Autodesk Inventor part; units mm, degrees
ref_plane "YZ Plane" through (0, 0, 0) normal (1, 0, 0) x (0, 1, 0)
ref_plane "XZ Plane" through (0, 0, 0) normal (0, 1, 0) x (-1, 0, 0)
ref_plane "XY Plane" through (0, 0, 0) normal (0, 0, 1) x (1, 0, 0)
sketch "Sketch1" plane through (0, 0, 0) normal (0, 1, 0) x (-1, 0, 0)
  line L0 (13.5, 10) -> (-13.5, 10)
  line L1 (-13.5, 10) -> (-13.5, -10)
  line L2 (-13.5, -10) -> (13.5, -10)
  line L3 (13.5, -10) -> (13.5, 10)
  line L4 (13.5, 10) -> (-13.5, -10) construction
  line L5 (-13.5, 10) -> (13.5, -10) construction
  point P0 (0, 0)
  dimension "d0" = 27
  dimension "d1" = 20
extrude "Extrusion1" add sketch "Sketch1" along normal blind 3
sketch "Sketch2" plane through (0, 3, 0) normal (0, 1, 0) x (1, 0, 0)
  line L0 (-13.5, -10) -> (13.5, -10)
  line L1 (0, -10) -> (-10.5, -10)
  line L2 (-10.5, -10) -> (-10.5, -7)
  line L3 (-10.5, -7) -> (-10.5, 3.5)
  circle A0 centre (-10.5, -7) radius 1.25
  circle A1 centre (-10.5, 3.5) radius 1.25
  line L4 (-10.5, -7) -> (10.5, -7)
  line L5 (10.5, -7) -> (10.5, 3.5)
  circle A2 centre (10.5, -7) radius 1.25
  circle A3 centre (10.5, 3.5) radius 1.25
  point P0 (0, 0)
  dimension "d4" = 10.5
  dimension "d5" = 3
  dimension "d6" = 10.5
  dimension "d7" = 2.5
  dimension "d8" = 2.5
  dimension "d9" = 21
  dimension "d10" = 10.5
  dimension "d11" = 2.5
  dimension "d12" = 2.5
extrude "Extrusion2" cut sketch "Sketch2" against normal up to next
sketch "Sketch3" plane through (0, 0, 0) normal (0, -1, 0) x (1, 0, 0)
  line L0 (-13.5, 10) -> (13.5, 10)
  line L1 (0, 10) -> (0, 8.5)
  line L2 (7.5, 7) -> (-7.5, 7)
  line L3 (-7.5, 7) -> (-7.5, 10)
  line L4 (-7.5, 10) -> (7.5, 10)
  line L5 (7.5, 10) -> (7.5, 7)
  line L6 (7.5, 7) -> (-7.5, 10) construction
  line L7 (-7.5, 7) -> (7.5, 10) construction
  point P0 (0, 0)
  dimension "d15" = 1.5
  dimension "d16" = 15
  dimension "d17" = 3
extrude "Extrusion3" add sketch "Sketch3" along normal blind 8
sketch "Sketch4" plane through (7.5, 0, 7) normal (0, 0, -1) x (-1, 0, 0)
  circle A0 centre (3, -5) radius 1.25
  circle A1 centre (12, -5) radius 1.25
  line L0 (0, 0) -> (0, -8)
  line L1 (15, -8) -> (0, -8)
  line L2 (15, 0) -> (15, -8)
  point P0 (7.5, 0)
  dimension "d20" = 2.5
  dimension "d21" = 2.5
  dimension "d22" = 3
  dimension "d23" = 3
  dimension "d24" = 3
  dimension "d25" = 3
extrude "Extrusion4" cut sketch "Sketch4" against normal up to next
sketch "Sketch5" plane through (0, 0, 0) normal (0, -1, 0) x (1, 0, 0)
  line L0 (13.5, -10) -> (-13.5, -10)
  line L1 (13.5, -10) -> (7.5, -10)
  line L2 (7.5, -10) -> (-7.5, -10)
  line L3 (-7.5, -10) -> (-7.5, 7)
  line L4 (-7.5, 7) -> (7.5, 7)
  line L5 (7.5, 7) -> (7.5, -10)
  point P0 (0, 0)
  dimension "d28" = 6
extrude "Extrusion5" cut sketch "Sketch5" against normal up to next
fillet "Fillet1" radius 5 2 edges at (-7.5, 1.5, 7) (7.5, 1.5, 7)
fillet "Fillet2" radius 3 10 edges at (7.5, 1.5, -10) (13.5, 1.5, -10) (-7.5, 1.5, -10) (-13.5, 1.5, -10) (-13.5, 1.5, 10) (13.5, 1.5, 10) (-7.5, -8, 8.5) (7.5, -8, 8.5) (-5, 0, 7) (5, 0, 7)
properties part number "cam_holder" material "Nylon 6/6"
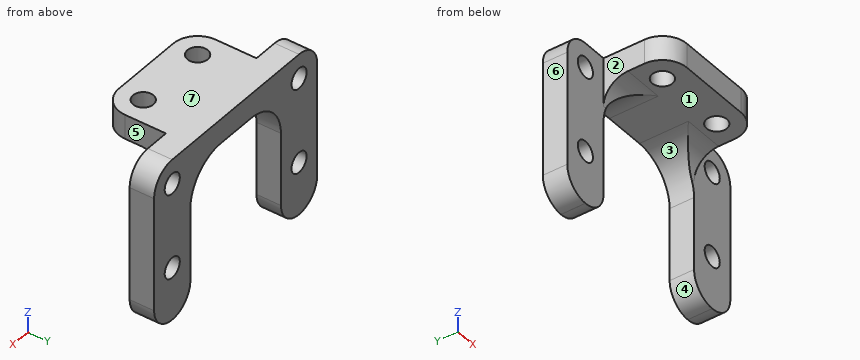
Check sheet for the modelled part. Datum: model origin and axes. Units: mm. Face numbers are marked on the shaded views. A direction names the side the tool comes from. Coordinates: 2 decimals unless noted, no trailing zeros. Loops run counter-clockwise (first coordinate to the right, second up) from the corner with the lowest first, then second, coordinate; pieces in that order, holes last. Notation, with made-up numbers: M 60,-26 L 67,-26 A10 ccw 67,-22 Z; hole C 7.25,27 d2. An arc over 180 degrees is marked long. Answer as a JSON object with one key per item and string values.
1. Depth check by flat-ended pin: P1, Ø3, axis at x = -9.5, z = -1, coming from the -Y side; P2, Ø1.5, axis at x = -7.5, y = -2, coming from the -Z side; P3, Ø3, axis at x = -4.5, y = -5, coming from the -Z side. Enter the tip coordinate at first touch or a pass-through.
Outcome:
{"P1": "y = 0", "P2": "z = 6.44", "P3": "z = 7"}
2. Release check for a two-part mould opening along X. For the marked faces 4, 5, 6 and 7 record: pulls with the +X half, pulls with the -X half, needs draft (parallel to the pull), parting line crosses it, or undercut.
Outcome:
{"face 4": "undercut", "face 5": "pulls with the +X half", "face 6": "pulls with the -X half", "face 7": "needs draft"}
3. Scan lines: L1, parallel to X at y = 1.7, z = -3.5; L2, parallel to Z at x = -10.5, y = 1.55; L3, parallel to Z at x = 11.5, y = 0.5. Record each from-to range of solid material in increasing order. Write a range as from..to.
Outcome:
{"L1": "-13.5..-11.75, -9.25..-7.5, 7.5..9.25, 11.75..13.5", "L2": "-10..-4.75, -2.25..5.75, 8.25..10", "L3": "-9.83..-4.25, -2.75..6.25, 7.75..9.83"}
4. Sectioned sample at D-D on x = 6.5. Record the cut outline in (y, z).
Outcome:
{"outline": "M -7.24,7 L -3,7 A3 cw -0.17,5 L 3,5 L 3,10 L -7.24,10 Z"}
5. Sectioned sample at A-A on z = 1. Record the cut outline in (x, y), and give its area (3 significant figures).
Outcome:
{"outline": "M -13.5,0 L -7.5,0 L -7.5,3 L -13.5,3 Z; M 7.5,0 L 13.5,0 L 13.5,3 L 7.5,3 Z", "area": "36.0 mm²"}
6. Sectioned sample at C-C on y = -1.5. Record the cut outline in (x, z), and give its area (3 significant figures).
Outcome:
{"outline": "M -7.5,6.6 L -4.46,6.6 A5 cw -2.5,7 L 2.5,7 A5 cw 4.46,6.6 L 7.5,6.6 L 7.5,10 L -7.5,10 Z", "area": "48.0 mm²"}
7. Sectioned sample at B-B on x = -5. Record the cut outline in (y, z).
Outcome:
{"outline": "M -7.96,7 L -6.15,7 L -6.15,10 L -7.96,10 Z; M -3.85,7 L -3,7 A3 cw -1.11,6.33 L 3,6.33 L 3,10 L -3.85,10 Z"}
8. Access from +Z, -Z, +X, -X, +Y, -Y to the whole of each face (thin tool, end or side, straight path). Record for the marked faces 1, 2 and 3.
Outcome:
{"face 1": "-Z, -Y", "face 2": "+Z, -Z, -X, -Y", "face 3": "-Z, +Y, -Y"}
